Could you check a few things on this model? Use its own coordinates, in mm. A direction names the side the tool comes from. Give positions to 0.01 mm unless a question says otherwise; leave off trailing zeros. Write each loop counter-clockwise with the first axis right and the second up, starting at its lowest first coordinate (ties: lowest second). Pieces come first, ordered by that corner, then holes. Notation, with made-up numbers: M -12,27 L 29,27 A24 cw 29,66 Z; hole C 78,72 d8. An arc over 180 degrees is marked long. Use one line per item in the form item = value.
from build123d import *

# Parameters (mm, degrees)
F1_DEPTH = 3.175
F0_W     = 13.9460621893
F0_H     = 3.175
F2_DEPTH = 19.05
F4_R     = 1.6002
F5_D     = 0.7874


with BuildPart() as f1:
    # F0 (on Top) → F1 (new body)
    with BuildSketch(Plane.XY):
        with BuildLine():
            ThreePointArc((-11.0640807489, -15.5076954182), (-10.5456846438, -17.739643222), (-8.337274974, -17.1286994839))
            ThreePointArc((-8.337274974, -17.1286994839), (-8.6896408656, -16.9526588365), (-9.0382916673, -16.7693704037))
            ThreePointArc((-9.0382916673, -16.7693704037), (-10.1433262143, -17.0628076037), (-10.4134929787, -15.9518545625))
            ThreePointArc((-10.4134929787, -15.9518545625), (-10.7410829362, -15.7331381917), (-11.0640807489, -15.5076954182))
        make_face()
        with BuildLine():
            ThreePointArc((-18.1676837587, 5.7304246652), (-20.1301990553, 4.5476908695), (-18.8667209135, 2.6361604601))
            ThreePointArc((-18.8667209135, 2.6361604601), (-18.8081833575, 3.0256798892), (-18.7416047219, 3.4139057466))
            ThreePointArc((-18.7416047219, 3.4139057466), (-19.3621545375, 4.3741789717), (-18.3890615299, 4.9744262032))
            ThreePointArc((-18.3890615299, 4.9744262032), (-18.2822807642, 5.3535698425), (-18.1676837587, 5.7304246652))
        make_face()
        with BuildLine():
            ThreePointArc((-0.9515720679, 19.0262190306), (-0.557987968, 19.0418263154), (-0.1641653109, 19.0492926312))
            ThreePointArc((-0.1641653109, 19.0492926312), (-1.8954625727, 20.5502707497), (-3.3229998068, 18.757936248))
            ThreePointArc((-3.3229998068, 18.757936248), (-2.934455716, 18.8226318471), (-2.5446570546, 18.8792801895))
            ThreePointArc((-2.5446570546, 18.8792801895), (-1.8231433853, 19.7661988811), (-0.9515720679, 19.0262190306))
        make_face()
        with BuildLine():
            ThreePointArc((17.8009576491, 6.7844238351), (17.9374252347, 6.4149260284), (18.0662240168, 6.0426856425))
            ThreePointArc((18.0662240168, 6.0426856425), (18.958738761, 8.1530749318), (16.8129940883, 8.9568817))
            ThreePointArc((16.8129940883, 8.9568817), (16.9945899865, 8.6073463501), (17.1689201725, 8.2541310937))
            ThreePointArc((17.1689201725, 8.2541310937), (17.9333659324, 8.1987289698), (18.3004742409, 7.5259153217))
            ThreePointArc((18.3004742409, 7.5259153217), (18.1639466917, 7.0788900287), (17.8009576491, 6.7844238351))
        make_face()
        with BuildLine():
            Line((0, -19.05), (0, 0))
            Line((0, 0), (2.5519689053, 0))
            Line((2.5519689053, 0), (2.5519689053, 3.175))
            Line((2.5519689053, 3.175), (16.4980310947, 3.175))
            Line((16.4980310947, 3.175), (16.4980310947, 0))
            Line((16.4980310947, 0), (19.05, 0))
            ThreePointArc((19.05, 0), (18.8024475471, 3.061121729), (18.0662240168, 6.0426856425))
            ThreePointArc((18.0662240168, 6.0426856425), (17.9374252347, 6.4149260284), (17.8009576491, 6.7844238351))
            ThreePointArc((17.8009576491, 6.7844238351), (16.7653585228, 7.2098268782), (17.1689201725, 8.2541310937))
            ThreePointArc((17.1689201725, 8.2541310937), (16.9945899865, 8.6073463501), (16.8129940883, 8.9568817))
            ThreePointArc((16.8129940883, 8.9568817), (9.7344781327, 16.3750552819), (-0.1641653109, 19.0492926312))
            ThreePointArc((-0.1641653109, 19.0492926312), (-0.557987968, 19.0418263154), (-0.9515720679, 19.0262190306))
            ThreePointArc((-0.9515720679, 19.0262190306), (-0.9500614951, 18.9978677335), (-0.9495577594, 18.969480692))
            ThreePointArc((-0.9495577594, 18.969480692), (-1.7044854564, 18.170656886), (-2.5446570546, 18.8792801895))
            ThreePointArc((-2.5446570546, 18.8792801895), (-2.934455716, 18.8226318471), (-3.3229998068, 18.757936248))
            ThreePointArc((-3.3229998068, 18.757936248), (-12.5654838561, 14.3182092268), (-18.1676837587, 5.7304246652))
            ThreePointArc((-18.1676837587, 5.7304246652), (-18.2822807642, 5.3535698425), (-18.3890615299, 4.9744262032))
            ThreePointArc((-18.3890615299, 4.9744262032), (-17.9515207228, 4.6908249859), (-17.7816222049, 4.1978684949))
            ThreePointArc((-17.7816222049, 4.1978684949), (-18.0756401917, 3.5781580739), (-18.7416047219, 3.4139057466))
            ThreePointArc((-18.7416047219, 3.4139057466), (-18.8081833575, 3.0256798892), (-18.8667209135, 2.6361604601))
            ThreePointArc((-18.8667209135, 2.6361604601), (-17.5003742409, -7.5259153217), (-11.0640807489, -15.5076954182))
            ThreePointArc((-11.0640807489, -15.5076954182), (-10.7410829362, -15.7331381917), (-10.4134929787, -15.9518545625))
            ThreePointArc((-10.4134929787, -15.9518545625), (-9.5143869792, -15.6058219661), (-8.9343781327, -16.3750552819))
            ThreePointArc((-8.9343781327, -16.3750552819), (-8.9607925373, -16.5789440003), (-9.0382916673, -16.7693704037))
            ThreePointArc((-9.0382916673, -16.7693704037), (-8.6896408656, -16.9526588365), (-8.337274974, -17.1286994839))
            ThreePointArc((-8.337274974, -17.1286994839), (-4.2778952087, -18.5634617619), (0, -19.05))
        make_face()
    extrude(amount=F1_DEPTH)

    # F0 (on Top) → F2 (join)
    with BuildSketch(Plane.XY):
        with Locations((9.525, 1.5875)):
            Rectangle(F0_W, F0_H)
    extrude(amount=F2_DEPTH)

    # F4
    f4_edges = [f1.edges().sort_by_distance(p)[0] for p in [
        (2.551969, 1.5875, 19.05),
        (16.498031, 1.5875, 19.05),
    ]]
    fillet(f4_edges, radius=F4_R)

    # F5 (through all)
    with Locations(Plane(origin=(0, 3.175, 0), x_dir=(-1, 0, 0), z_dir=(0, 1, 0))):
        with Locations((-3.8969237357, 18.2043871596), (-15.1530762643, 18.2043871596)):
            Hole(F5_D / 2)


solid = f1.part
1) For faces 5 (the cylindrical face through (18.81, 3.02, 1.57)), 6 (the flat face through (16.498, 2, 10)), 7 (the flat face through (2.552, 2, 10)), 8 (the cylindrical face through (-4.34, -18.55, 1.57)), which set-ups out of +Z, -Z, +X, -X, +Y, -Y let a thin tool reach every point of the face, with its end or its side?
Checked values:
face_5 = +Z, -Z, +X
face_6 = +Z, +X, +Y, -Y
face_7 = +Z, -X, +Y, -Y
face_8 = +Z, -Z, -Y
2) I want a section at B-B, the plane z = 8.25. Please give me the cut outline in (x, y) (3 decimals), plus the area to 3 significant figures.
Checked values:
outline = M 2.552,0 L 16.498,0 L 16.498,3.175 L 2.552,3.175 Z
area = 44.3 mm2
3) Thinking about a two-plate mould opening in Y: for faces 1 (the flat face through (0, -10, 2)), 2 (the cylindrical face through (9.86, 16.3, 1.57)), 3 (the flat face through (9, 0, 9)), 4 (the cylindrical face through (-10.58, -17.72, 1.57)), which applies, released by +Y, released by -Y, zero draft, split by the parting line, or undercut?
Checked values:
face_1 = zero draft
face_2 = released by +Y
face_3 = released by -Y
face_4 = undercut
4) For pin 1 Ø1.6 at (y, z) = (1.5, 10.5) entering from -X; pin 2 Ø1.5 at (x, z) = (12, 13.5) entering from -Y; pin 3 Ø8 at (x, y) = (1, -10.5) entering from +Z (3 decimals), each with a flat end and sliding along its axis, tell me the tip position at first contact or that it passes through.
Checked values:
pin_1 = 2.55
pin_2 = 0
pin_3 = 3.175
5) I want a section at C-C, the plane y = 13.5. Please give me the cut outline in (x, z) (3 decimals).
Checked values:
outline = M -13.441,0 L 13.441,0 L 13.441,3.175 L -13.441,3.175 Z
6) I want a section at A-A, the plane x = 7. Please give me the cut outline in (y, z) (3 decimals), plus the area to 3 significant figures.
Checked values:
outline = M 0,0 L 17.717,0 L 17.717,3.175 L 3.175,3.175 L 3.175,19.05 L 0,19.05 Z
area = 107 mm2
7) I want a section at D-D, the plane x = 13.5. Please give me the cut outline in (y, z) (3 decimals).
Checked values:
outline = M 0,0 L 13.441,0 L 13.441,3.175 L 3.175,3.175 L 3.175,19.05 L 0,19.05 Z
8) If I drill on L1, parallel to Z at x = 9, y = 7 (3 decimals); L2, parallel to Y at x = -1.5, z = 1.25, over which ranges is the centre line in solid material (lowest first)?
Checked values:
L1 = 0 to 3.175
L2 = -18.99 to 18.21, 19.73 to 20.54
